Input: part model. Units: mm. Frame: model coordinates. A direction names the side the tool comes from. Give positions to 0.01 mm unless a question says otherwise; leave off trailing zeros. Write each loop counter-clockwise with the first axis right and the second up, starting at its lowest first coordinate (ties: lowest second). Pieces come first, ordered by that corner, then holes.
```python
from build123d import *

# Parameters (mm, degrees)
F2_R          = 0.381
F3_SIZE       = 0.381
F4_SIZE       = 0.7874
F5_SIZE2      = 0.9092112039
F5_SIZE       = 1.5748
F7_DEPTH      = 84.1385
F7_DEPTH_BACK = 84.1385
F8_SIZE       = 0.381
F11_DEPTH     = 15.875
F12_R         = 7.9375
F13_R         = 7.93749


# Not quite as in the source:
# - a fillet or chamfer is up to 0.001 mm smaller than in the source, because OpenCascade refuses the exact size


with BuildPart() as f1:
    # F0 (on Right) → F1 (revolve)
    with BuildSketch(Plane.YZ):
        Polygon((84.1375, -4.5212), (84.1375, 0), (69.0626, 0), (69.0626, -60.325), (63.8937, -69.2777974192), (63.8937, -92.075), (80.9625, -92.075), (80.9625, -4.5212), align=None)
    revolve(axis=Axis((0, 0, -46.0375), (0, 0, -1)))

    # F2
    f2_edges = [f1.edges().sort_by_distance(p)[0] for p in [
        (0, -80.9625, -4.5212),
    ]]
    fillet(f2_edges, radius=F2_R)

    # F3
    f3_edges = [f1.edges().sort_by_distance(p)[0] for p in [
        (0, -84.1375, -4.5212),
        (0, -84.1375, 0),
        (0, 84.1375, -2.2606),
    ]]
    chamfer(f3_edges, length=F3_SIZE)

    # F4
    f4_edges = [f1.edges().sort_by_distance(p)[0] for p in [
        (0, -69.0626, 0),
    ]]
    chamfer(f4_edges, length=F4_SIZE)

    # F5
    f5_edges = [f1.edges().sort_by_distance(p)[0] for p in [
        (0, -63.8937, -92.075),
    ]]
    chamfer(f5_edges, length=F5_SIZE, length2=F5_SIZE2)

    # F6 (on Right) → F7 (cut, two sides)
    with BuildSketch(Plane.YZ) as f7_sk:
        Polygon((-80.9625, -74.6285183865), (-80.9625, -92.075), (-74.6125, -92.075), align=None)
    extrude(amount=F7_DEPTH, mode=Mode.SUBTRACT)
    extrude(f7_sk.sketch, amount=-F7_DEPTH_BACK, mode=Mode.SUBTRACT)

    # F8
    f8_edges = [f1.edges().sort_by_distance(p)[0] for p in [
        (79.359123, 16.032964, -92.075),
    ]]
    chamfer(f8_edges, length=F8_SIZE)

    # F10 (on offset) → F11 (cut)
    with BuildSketch(Plane.XY.offset(-31.75)):
        with BuildLine():
            Line((-39.6126799931, -56.5727699739), (-46.4381822281, -66.3205973857))
            ThreePointArc((-46.4381822281, -66.3205973857), (0, -80.9625), (46.4381822281, -66.3205973857))
            Line((46.4381822281, -66.3205973857), (39.6126799931, -56.5727699739))
            ThreePointArc((39.6126799931, -56.5727699739), (0, -69.0626), (-39.6126799931, -56.5727699739))
        make_face()
    extrude(amount=-F11_DEPTH, mode=Mode.SUBTRACT)

    # F12
    f12_edges = [f1.edges().sort_by_distance(p)[0] for p in [
        (-43.025431, -61.446684, -31.75),
        (43.025431, -61.446684, -31.75),
    ]]
    fillet(f12_edges, radius=F12_R)

    # F13 (radius 7.9375 in the source; OpenCascade refuses exactly that, so slightly less here)
    f13_edges = [f1.edges().sort_by_distance(p)[0] for p in [
        (-43.025431, -61.446684, -47.625),
        (43.025431, -61.446684, -47.625),
    ]]
    fillet(f13_edges, radius=F13_R)


solid = f1.part
```
Q1. Pin query (flat end, axial travel): pin 1 (4 mm diameter, centred on x = 11.5, z = -70, fed in from +Y); pin 2 (2 mm diameter, centred on x = 61, y = 49.5, fed in from +Z); pin 3 (5 mm diameter, centred on x = 5.5, z = -74.5, fed in from +Y); pin 4 (3 mm diameter, centred on x = -18.5, z = -67, fed in from -Y). Return the tip coordinate at first contact, or that it passes through.
Q2. Section C-C, the plane z = -22.5. Return the cut outline in (x, y) (1 decimal), then the cut area to 3 significant figures.
Q3. Mould query, pull axis Y, two halves, no side actions, for faces 1 (the flat face through (-1, -73, -31.75)), 2 (the flat face through (-0.44, -77.04, -85.41)), 3 (the conical face through (19.3, 61.2, -68.8)), 4 (the cylindrical face through (24.319, 77.224, -47.691)). Classes: +Y half, -Y half, draft (parallel to the pull), parting line (faces both ways), or undercut.
Q4. Material intervals for line 1 along X through (y, z) = (0, -75); line 2 along X through (y, z) = (0, -23); line 3 along Y through (x, z) = (0, -47.5), sorted ascending.
Q5. Section D-D, the plane z = -43. Return the cut outline in (x, y) (1 decimal).
Q6. Section A-A, the plane x = 0. Give the number of separate pieces and of enclosed holes in the cut face, then the cut area to 3 significant figures.
Q7. Access query for faces 5 (the cylindrical face through (20.745, 65.873, -30.973)), 6 (the flat face through (44, 69, -4.521)), 7 (the cylindrical face through (-40.989, -62.699, -34.013)). Directions: +Z, -Z, +X, -X, +Y, -Y. A direction counts if a zero-diameter tool reaches every point of the face in a straight line with its end or side. Return the directions, or none.
Solutions:
1. pin 1: stops at y = 80.4
1. pin 2: stops at z = 0
1. pin 3: stops at y = 80.91
1. pin 4: stops at y = -79.16
2. outline: circle Ø161.9 at (0, 0); hole circle Ø138.1 at (0, 0)
2. area: 5,610 mm2
3. face 1: draft
3. face 2: -Y half
3. face 3: undercut
3. face 4: parting line
4. line 1: x = -80.96 to -63.89, 63.89 to 80.96
4. line 2: x = -80.96 to -69.06, 69.06 to 80.96
4. line 3: y = 69.06 to 80.96
5. outline: (-45.8, -66.7) - (-39, -57) arc R69.1 cw (long way) to (39, -57) - (45.8, -66.7) arc R81 ccw (long way) to start
6. separate pieces: 3
6. enclosed holes: 0
6. area: 2,260 mm2
7. face 5: +Z
7. face 6: -Z
7. face 7: -Y
